Source: CAD feature listing. Evaluate the final solid. Frame: model axes, mm. Round coordinates to 2 decimals unless told otherwise and drop trailing zeros. Loops run counter-clockwise (first coordinate to the right, second up) from the corner with the lowest first, then second, coordinate; pieces in that order, holes last. Notation, with made-up numbers: M 69.5,71.25 L 87.5,71.25 A18 cw 87.5,97.25 Z; hole C 7,84 d1. An arc over 180 degrees is marked long. Write each question's results on one line, items separated by ' | '. Start each with the question number.
1. Contact query for flat-ended pins moving along their axis: pin 1 Ø2 at (x, z) = (-45.5, -2) entering from -Y; pin 2 Ø3 at (y, z) = (1, -2.5) entering from -X; pin 3 Ø3 at (y, z) = (-12.5, -5.5) entering from +X. Output: stop coordinate, or through.
2. Section A-A on y = 20. Output: boundary loops of the cut face in (x, z).
3. Section C-C on x = -21. Output: boundary loops of the cut face in (y, z).
4. Ray query, line 1 (X direction, y = 20.5, z = -4.6); line 2 (X direction, y = 1, z = -5); line 3 (Y direction, x = -37, z = -4.85). Return the intervals inside material, ascending.
5. Section D-D on y = 6. Output: boundary loops of the cut face in (x, z), and give its area (3 significant figures).
from build123d import *

# Parameters (mm, degrees)
ESQUISSE1_W             = 151
ESQUISSE1_H             = 54
ESQUISSE1_W_2           = 101
ESQUISSE1_H_2           = 19
BOSS_EXTRU_1_DEPTH      = 6
ESQUISSE2_W             = 10
ESQUISSE2_H             = 32
ENL_V_MAT_EXTRU_1_DEPTH = 6
ESQUISSE4_W             = 32
ESQUISSE4_H             = 10
ENL_V_MAT_EXTRU_2_DEPTH = 10


with BuildPart() as part:
    # Esquisse1 → Boss.-Extru.1 (new body)
    with BuildSketch(Plane.XY):
        Rectangle(ESQUISSE1_W, ESQUISSE1_H)
        Rectangle(ESQUISSE1_W_2, ESQUISSE1_H_2, mode=Mode.SUBTRACT)
    extrude(amount=-BOSS_EXTRU_1_DEPTH)

    # Esquisse2 → Enlèv. mat.-Extru.1 (cut)
    with BuildSketch(Plane.XY):
        with Locations((-70.5, 0)):
            Rectangle(ESQUISSE2_W, ESQUISSE2_H)
        with Locations((70.5, 0)):
            Rectangle(ESQUISSE2_W, ESQUISSE2_H)
    extrude(amount=-ENL_V_MAT_EXTRU_1_DEPTH, mode=Mode.SUBTRACT)

    # Esquisse4 → Enlèv. mat.-Extru.2 (cut)
    with BuildSketch(Plane.XY):
        with Locations((33, 22)):
            Rectangle(ESQUISSE4_W, ESQUISSE4_H)
        with Locations((-33, 22)):
            Rectangle(ESQUISSE4_W, ESQUISSE4_H)
        with Locations((-33, -22)):
            Rectangle(ESQUISSE4_W, ESQUISSE4_H)
        with Locations((33, -22)):
            Rectangle(ESQUISSE4_W, ESQUISSE4_H)
    extrude(amount=-ENL_V_MAT_EXTRU_2_DEPTH, mode=Mode.SUBTRACT)


solid = part.part
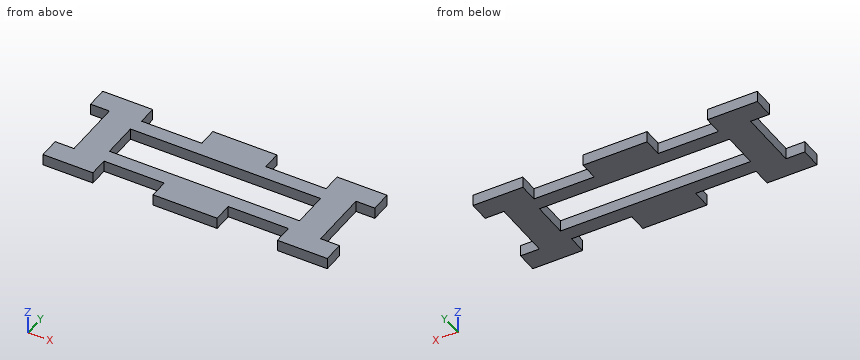
Taken from the geometry:
1) pin 1: y = -17 | pin 2: x = -65.5 | pin 3: x = 65.5
2) outline: M -75.5,-6 L -49,-6 L -49,0 L -75.5,0 Z; M -17,-6 L 17,-6 L 17,0 L -17,0 Z; M 49,-6 L 75.5,-6 L 75.5,0 L 49,0 Z
3) outline: M -17,-6 L -9.5,-6 L -9.5,0 L -17,0 Z; M 9.5,-6 L 17,-6 L 17,0 L 9.5,0 Z
4) line 1: -75.5 to -49, -17 to 17, 49 to 75.5 | line 2: -65.5 to -50.5, 50.5 to 65.5 | line 3: -17 to -9.5, 9.5 to 17
5) outline: M -65.5,-6 L -50.5,-6 L -50.5,0 L -65.5,0 Z; M 50.5,-6 L 65.5,-6 L 65.5,0 L 50.5,0 Z | area: 180 mm^2
